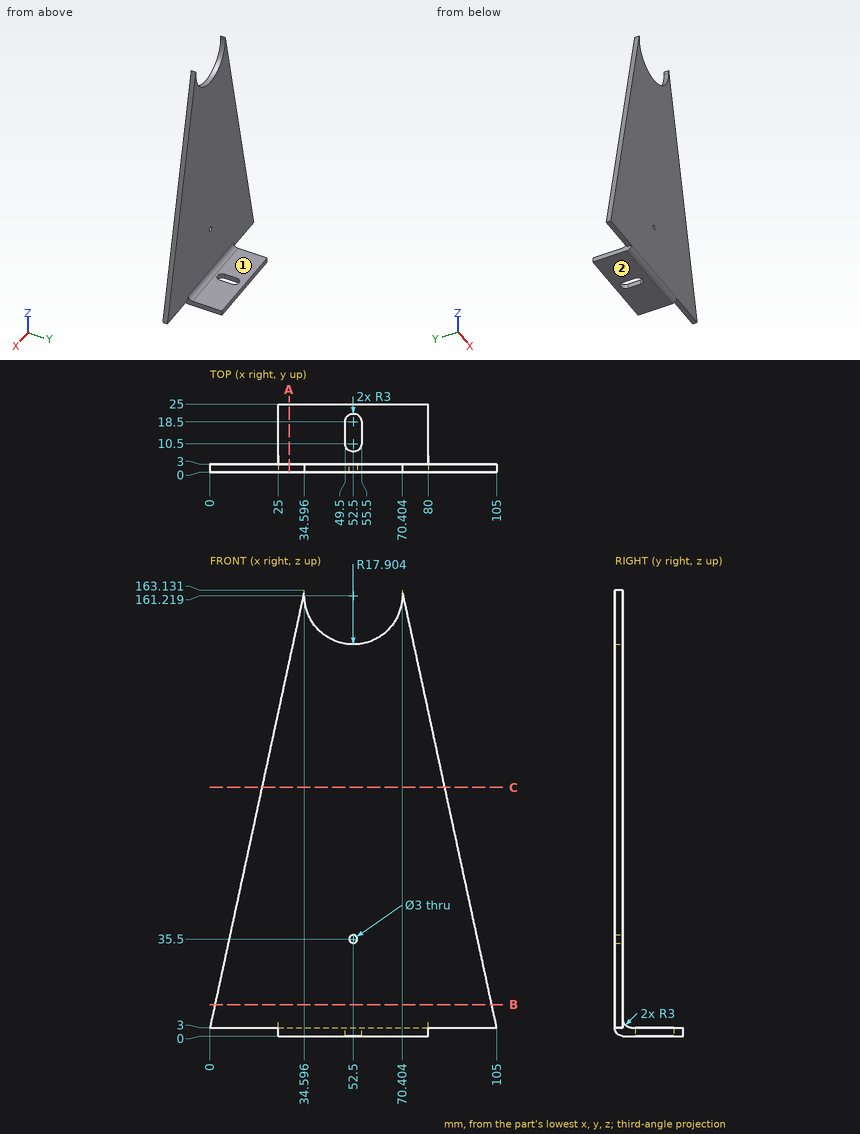
Geometry check sheet. Reference: drawing and pictorial views, mm from the part's lowest x, y, z. A direction names the side the tool comes from. Coordinates: 2 decimals unless noted, no trailing zeros. Order: outer loops, then holes, each group sorted by start corner. A loop starts at its lowest first (then second) coordinate and runs counter-clockwise, first axis right, second up. Notation, with made-up numbers: (-20, 41) -> (15, 41) arc R25 cw to (15, 68) -> close; hole circle Ø1 at (57.5, -20.75). An arc over 180 degrees is marked (long way). Put each result on its own line as item: value. Start each with the question number.
1) Go/stop test with flat-tipped pins: pin 1 (10 mm diameter, centred on y = 2.5, z = 64.5, fed in from +X); pin 2 (1.8 mm diameter, centred on y = 7.5, z = 2.5, fed in from -X); pin 3 (3 mm diameter, centred on y = 18, z = 2, fed in from +X); pin 4 (1.8 mm diameter, centred on x = 52.5, z = 35.5, fed in from +Y). Record where each tip stops, or that it passes through.
2) Material ranges on L1, parallel to Y at x = 85.5, z = 56; L2, parallel to Z at x = 52.5, y = 1.1 (1 decimal), recorded low to high.
3) Tool access check on the marked faces 1 and 2. Record the directions out of +Z, -Z, +X, -X, +Y, -Y that give a thin tool (end or side, any length) a straight path to the whole face; none if there is none.
4) Cross-section at A-A (x = 29). Enter the section's corners in (y, z), plus the area to 3 significant figures.
5) Cross-section at C-C (z = 91). Enter the section's corners in (x, y).
6) Cross-section at B-B (z = 11.5). Enter the section's corners in (x, y).
Geometry check:
1. pin 1: stops at x = 92.79
1. pin 2: stops at x = 25
1. pin 3: stops at x = 80
1. pin 4: passes through
2. L1: y = 0 to 3
2. L2: z = 0.7 to 34, 37 to 143.3
3. face 1: +Z, +X, -X, +Y
3. face 2: -Z, +X, -X, +Y, -Y
4. outline: (0, 3) arc R3 ccw to (3, 0) -> (25, 0) -> (25, 3) -> (6, 3) arc R3 cw to (3, 6) -> (3, 137.23) -> (0, 137.23) -> close
4. area: 478 mm^2
5. outline: (19.01, 0) -> (85.99, 0) -> (85.99, 3) -> (19.01, 3) -> close
6. outline: (1.84, 0) -> (103.16, 0) -> (103.16, 3) -> (1.84, 3) -> close
